The figure shows three views and two pictorial views of one solid part (mm, origin at its lowest corner). Answer the questions. Round coordinates to 2 decimals unless told otherwise and drop trailing zeros. Write each loop counter-clockwise with the first axis right and the second up, starting at its lowest first coordinate (ties: lowest second). Pieces come first, ordered by that corner, then holes. Notation, with made-up numbers: M 45,11 L 73,11 A22 ccw 73,39 Z; hole C 52.25,51 d8. An arc over 180 degrees is marked long. Answer in a Markdown table with one row per item.
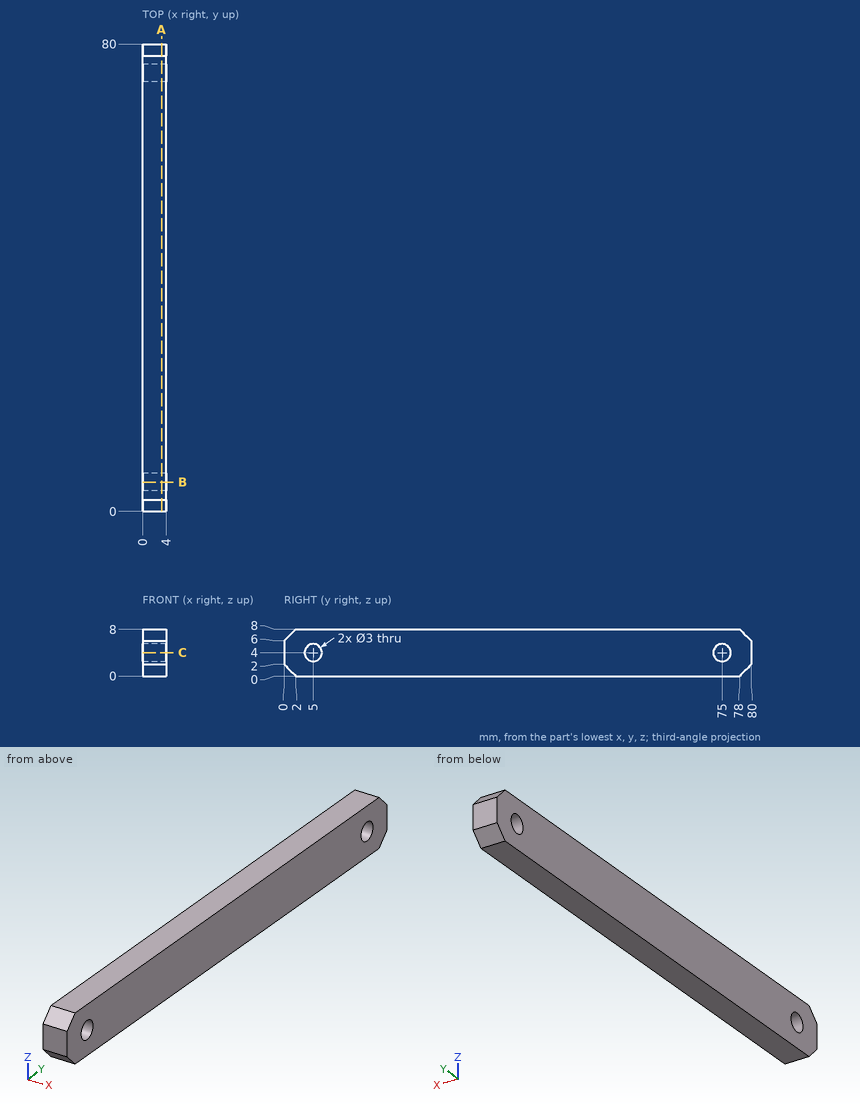
1. The part is cut by section A-A (x = 3.25). Determine the outline of the cut face in (y, z), plus the area to 3 significant figures.
Calculated:
| item | result |
|---|---|
| outline | M 0,2 L 2,0 L 78,0 L 80,2 L 80,6 L 78,8 L 2,8 L 0,6 Z; hole C 5,4 d3; hole C 75,4 d3 |
| area | 618 mm² |
2. The part is cut by section B-B (y = 5). Determine the outline of the cut face in (x, z), plus the area to 3 significant figures.
Calculated:
| item | result |
|---|---|
| outline | M 0,0 L 4,0 L 4,2.5 L 0,2.5 Z; M 0,5.5 L 4,5.5 L 4,8 L 0,8 Z |
| area | 20.0 mm² |
3. The part is cut by section C-C (z = 4). Determine the outline of the cut face in (x, y), plus the area to 3 significant figures.
Calculated:
| item | result |
|---|---|
| outline | M 0,0 L 4,0 L 4,3.5 L 0,3.5 Z; M 0,6.5 L 4,6.5 L 4,73.5 L 0,73.5 Z; M 0,76.5 L 4,76.5 L 4,80 L 0,80 Z |
| area | 296 mm² |
4. Consider line 1 along Y through (x, z) = (2.55, 4); line 2 along Z through (x, y) = (3.05, 75); line 3 along Y through (x, z) = (0.9, 5.25). Determine where each line is inside the solid, lowest interval first. Write a range as from..to.
Calculated:
| item | result |
|---|---|
| line 1 | y = 0..3.5, 6.5..73.5, 76.5..80 |
| line 2 | z = 0..2.5, 5.5..8 |
| line 3 | y = 0..4.17, 5.83..74.17, 75.83..80 |
